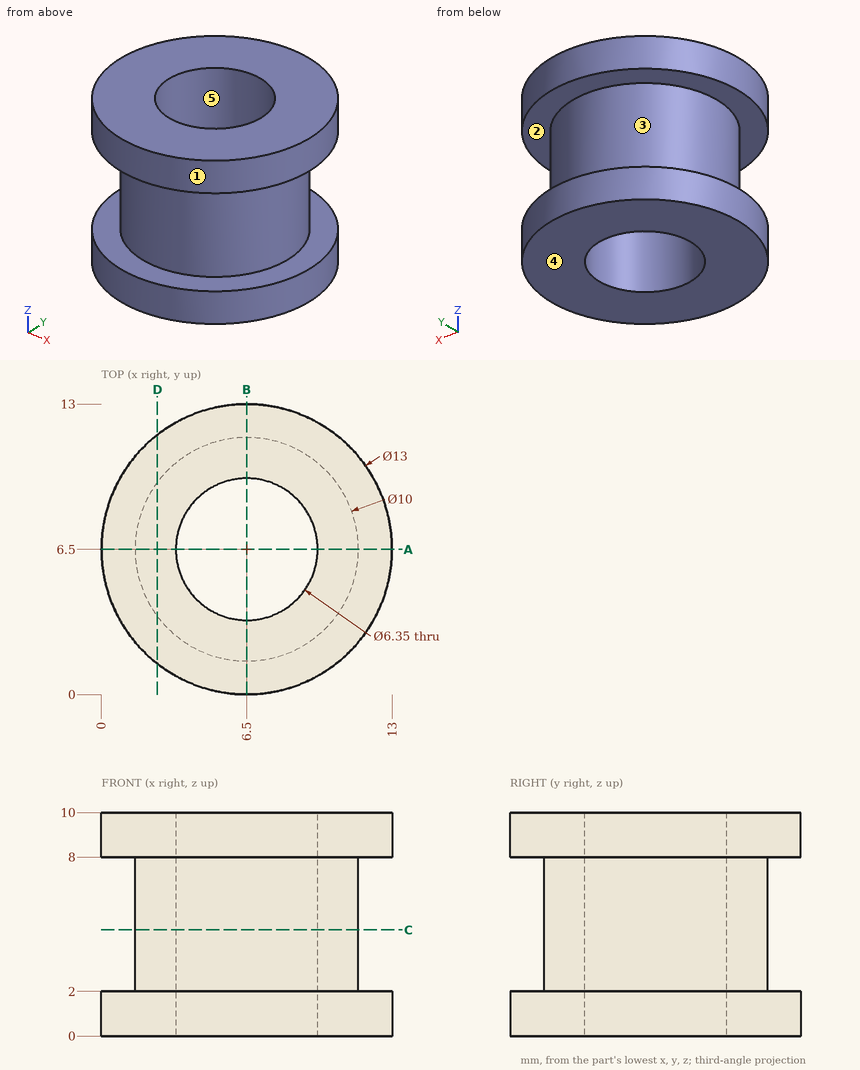
Design review of the part shown in the three views and the two pictorial views. Dimensions are in mm from the part's minimum x, y and z. A direction names the side the tool comes from. Coordinates: 2 decimals unless noted, no trailing zeros. Write each loop counter-clockwise with the first axis right and the second up, starting at its lowest first coordinate (ties: lowest second). Pieces come first, ordered by that corner, then holes. Notation, with made-up numbers: (32, -9) -> (70, -9) arc R10 ccw to (70, -2) -> close; hole circle Ø4 at (-21, 10.5). An arc over 180 degrees is marked (long way). Answer in a Markdown table with one row per item.
1. For the marked faces 1 and 2, list the 3-axis set-ups (+Z, -Z, +X, -X, +Y, -Y) from which the entire face can be reached by the end or side of a thin tool; tool diameter is ignored.
Answers below:
| item | result |
|---|---|
| face 1 | +Z, -Z |
| face 2 | none |
2. We need section A-A, the plane y = 6.5. State the section outline as (x, z) points (3 decimals), and give its area (3 significant figures).
Answers below:
| item | result |
|---|---|
| outline | (0, 0) -> (3.325, 0) -> (3.325, 10) -> (0, 10) -> (0, 8) -> (1.5, 8) -> (1.5, 2) -> (0, 2) -> close; (9.675, 0) -> (13, 0) -> (13, 2) -> (11.5, 2) -> (11.5, 8) -> (13, 8) -> (13, 10) -> (9.675, 10) -> close |
| area | 48.5 mm^2 |
3. We need section C-C, the plane z = 4.75. State the section outline as (x, y) points (3 decimals).
Answers below:
| item | result |
|---|---|
| outline | circle Ø10 at (6.5, 6.5); hole circle Ø6.35 at (6.5, 6.5) |
4. Clearance check with a flat-ended pin moving along its axis: pin 1 Ø1.5 at (x, z) = (9, 8.5) entering from +Y. State where the tip first meets the part, or that it passes through.
Answers below:
| item | result |
|---|---|
| pin 1 | stops at y = 12.76 |
5. Draft analysis for pull direction Y (two halves, no side actions). For the marked faces 3, 4 and 5, state which applies: +Y half, -Y half, draft (parallel to the pull), parting line (faces both ways), or undercut.
Answers below:
| item | result |
|---|---|
| face 3 | parting line |
| face 4 | draft |
| face 5 | undercut |
6. We need section D-D, the plane x = 2.5. State the section outline as (y, z) points, and give its area (3 significant figures).
Answers below:
| item | result |
|---|---|
| outline | (1.38, 0) -> (11.62, 0) -> (11.62, 2) -> (9.5, 2) -> (9.5, 8) -> (11.62, 8) -> (11.62, 10) -> (1.38, 10) -> (1.38, 8) -> (3.5, 8) -> (3.5, 2) -> (1.38, 2) -> close |
| area | 77.0 mm^2 |
7. Wall thickness on probe 1 along Z at (x, y) = (9.75, 2.5); probe 2 along Y at (x, z) = (6.5, 6.5) (3 decimals); probe 3 along Y at (x, z) = (4.5, 1.75): over which ranges is each line inside the solid? List them lowest first. Write a range as [from, to].
Answers below:
| item | result |
|---|---|
| probe 1 | z = [0, 2], [8, 10] |
| probe 2 | y = [1.5, 3.325], [9.675, 11.5] |
| probe 3 | y = [0.32, 4.03], [8.97, 12.68] |
